For this review, take the finished solid that the model builds, in its own axes (mm). A direction names the side the tool comes from. Coordinates: 2 decimals unless noted, no trailing zeros. Loops run counter-clockwise (first coordinate to the right, second up) from the corner with the lowest first, then second, coordinate; pieces in that order, holes last. Notation, with made-up numbers: (73, 88) - (119, 88) arc R18 cw to (119, 102) - close; hole circle Ø11 at (-28.75, 63.25). An arc over 180 degrees is marked (long way). Use one line per item in the form item = value. Start each with the question number.
1. Draft analysis for pull direction Y (two halves, no side actions). For faces 1 (the face through (10.441, 12.377, 2.958)), 2 (the face through (16.5, -12, 3)), 3 (the face through (-10, -10, 3)), state which applies: +Y half, -Y half, draft (parallel to the pull), parting line (faces both ways), or undercut.
2. Add section A-A on x = 12.5. Give the boundary of the cut face in (y, z).
3. Add section C-C on x = 26. Give the boundary of the cut face in (y, z), and give its area (3 significant figures).
4. To check wall thickness, follow probe 1 along Y at (x, z) = (12.5, 1.45); probe 2 along X at (y, z) = (-11.5, 2.35); probe 3 along Y at (x, z) = (5, 1.05). State the ranges of each line that lie inside material, in increasing order.
5. Machinability: for faces 4 (the face through (-7.5, -12, 3)), 5 (the face through (10, -10, 3)), 6 (the face through (0, 21, 3)), 7 (the face through (28.5, -13, 3)), which of the approach directions +Z, -Z, +X, -X, +Y, -Y give a long, thin tool a straight path to every point of the face, cutting with its end or side? Answer none if there is none.
6. For pin 1 Ø4 at (x, y) = (1.5, 5.5) entering from -Z; pin 2 Ø4 at (x, y) = (28.5, 5.5) entering from -Z; pin 3 Ø2.5 at (x, z) = (31, 2) entering from -Y; pin 4 Ø1 at (y, z) = (9, 1) entering from +X, all flat-tipped, find the tip position at first contact; note any pin that passes through.
7. Add section B-B on y = 14.5. Give the boundary of the cut face in (x, z), and give its area (3 significant figures).
```python
from build123d import *

# Parameters (mm, degrees)
CROQUIS1_R              = 9.5
SALIENTE_EXTRUIR1_DEPTH = 6


with BuildPart() as part:
    # Croquis1 → Saliente-Extruir1 (new body)
    with BuildSketch(Plane.XY):
        with BuildLine():
            Line((-12.5, 0), (-12.5, -10))
            Line((-12.5, -10), (-7.5, -10))
            Line((-7.5, -10), (-7.5, -15))
            Line((-7.5, -15), (4.5, -15))
            Line((4.5, -15), (4.5, -10))
            Line((4.5, -10), (16.5, -10))
            Line((16.5, -10), (16.5, -15))
            Line((16.5, -15), (28.5, -15))
            Line((28.5, -15), (28.5, -10))
            Line((28.5, -10), (33.5, -10))
            Line((33.5, -10), (24.60996669, 24.748813068))
            ThreePointArc((24.60996669, 24.748813068), (10.938683829, 34.052743456), (0, 21.650635095))
            Line((0, 21.650635095), (0, 20.155644371))
            ThreePointArc((0, 20.155644371), (-1.501634144, 14.885181604), (-5.555555556, 11.197580206))
            ThreePointArc((-5.555555556, 11.197580206), (-10.62295732, 6.588078459), (-12.5, 0))
        make_face()
        Circle(CROQUIS1_R, mode=Mode.SUBTRACT)
        with Locations((12.5, 21.650635095)):
            Circle(CROQUIS1_R, mode=Mode.SUBTRACT)
    extrude(amount=SALIENTE_EXTRUIR1_DEPTH)


solid = part.part
```
Conclusion:
q1.face_1 = undercut
q1.face_2 = draft
q1.face_3 = -Y half
q2.outline = (-10, 0) - (12.15, 0) - (12.15, 6) - (-10, 6) - close; (31.15, 0) - (34.15, 0) - (34.15, 6) - (31.15, 6) - close
q3.outline = (-15, 0) - (19.32, 0) - (19.32, 6) - (-15, 6) - close
q3.area = 206 mm^2
q4.probe_1 = -10 to 12.15, 31.15 to 34.15
q4.probe_2 = -7.5 to 4.5, 16.5 to 28.5
q4.probe_3 = -10 to -8.08, 8.08 to 15.82, 27.48 to 31.65
q5.face_4 = +Z, -Z, -X, -Y
q5.face_5 = +Z, -Z, -Y
q5.face_6 = +Z, -Z, -X, +Y
q5.face_7 = +Z, -Z, +X, -Y
q6.pin_1 = through
q6.pin_2 = 0
q6.pin_3 = -10
q6.pin_4 = 28.77
q7.outline = (-1.75, 0) - (6.25, 0) - (6.25, 6) - (-1.75, 6) - close; (18.75, 0) - (27.23, 0) - (27.23, 6) - (18.75, 6) - close
q7.area = 98.9 mm^2
